from build123d import *

# Parameters (mm, degrees)
BOSS_EXTRUDE1_DEPTH = 4
SKETCH2_R           = 6.5
SKETCH2_R_2         = 2.25
SKETCH2_R_3         = 4
CUT_EXTRUDE1_DEPTH  = 4
BOSS_EXTRUDE2_START = 4
SKETCH3_R           = 22
SKETCH3_R_2         = 19
BOSS_EXTRUDE2_DEPTH = 15
SKETCH4_R           = 13.1
SKETCH4_R_2         = 11.1
BOSS_EXTRUDE3_DEPTH = 10
SKETCH5_R           = 1.5
CUT_EXTRUDE2_DEPTH  = 103.505675922
SKETCH6_W           = 10
SKETCH6_H           = 40
CUT_EXTRUDE3_DEPTH  = 103.505675922
FILLET1_R           = 2


with BuildPart() as part:
    # Sketch1 → Boss-Extrude1 (new body)
    with BuildSketch(Plane.XY):
        with BuildLine():
            Line((-14.334769336, 37.652327005), (51.395230664, 37.652327005))
            ThreePointArc((51.395230664, 37.652327005), (91.395230664, -2.347672995), (51.395230664, -42.347672995))
            Line((51.395230664, -42.347672995), (-14.334769336, -42.347672995))
            ThreePointArc((-14.334769336, -42.347672995), (-54.334769336, -2.347672995), (-14.334769336, 37.652327005))
        make_face()
    extrude(amount=BOSS_EXTRUDE1_DEPTH)

    # Sketch2 → Cut-Extrude1 (cut)
    with BuildSketch(Plane.XY):
        with Locations(Location((44.395230664, -2.347672995, 0), (0, 0, 180))):
            Circle(SKETCH2_R)
        with Locations(Location((51.395230664, 13.152327005, 0), (0, 0, 180))):
            Circle(SKETCH2_R_2)
        with Locations(Location((64.818624423, 5.402327005, 0), (0, 0, 180))):
            Circle(SKETCH2_R_2)
        with Locations(Location((64.818624423, -10.097672995, 0), (0, 0, 180))):
            Circle(SKETCH2_R_2)
        with Locations(Location((51.395230664, -17.847672995, 0), (0, 0, 180))):
            Circle(SKETCH2_R_2)
        with Locations(Location((37.971836906, -10.097672995, 0), (0, 0, 180))):
            Circle(SKETCH2_R_2)
        with Locations(Location((37.971836906, 5.402327005, 0), (0, 0, 180))):
            Circle(SKETCH2_R_2)
        with Locations(Location((-14.334769336, -2.347672995, 0), (0, 0, 180))):
            Circle(SKETCH2_R_3)
    extrude(amount=CUT_EXTRUDE1_DEPTH, mode=Mode.SUBTRACT)

    # Sketch3 → Boss-Extrude2 (add)
    with BuildSketch(Plane.XY.offset(BOSS_EXTRUDE2_START)):
        with Locations(Location((51.395230664, -2.347672995, 0), (0, 0, 180))):
            Circle(SKETCH3_R)
        with Locations(Location((51.395230664, -2.347672995, 0), (0, 0, 180))):
            Circle(SKETCH3_R_2, mode=Mode.SUBTRACT)
    extrude(amount=BOSS_EXTRUDE2_DEPTH)

    # Sketch4 → Boss-Extrude3 (add)
    with BuildSketch(Plane.XY):
        with Locations(Location((-14.334769336, -2.347672995, 0), (0, 0, 180))):
            Circle(SKETCH4_R)
        with Locations(Location((-14.334769336, -2.347672995, 0), (0, 0, 180))):
            Circle(SKETCH4_R_2, mode=Mode.SUBTRACT)
    extrude(amount=BOSS_EXTRUDE3_DEPTH)

    # Sketch5 → Cut-Extrude2 (cut, through all)
    with BuildSketch(Plane.XY):
        with Locations(Location((88.395230664, -2.347672995, 0), (0, 0, 180))):
            Circle(SKETCH5_R)
        with Locations(Location((-51.334769336, -2.347672995, 0), (0, 0, 180))):
            Circle(SKETCH5_R)
        with Locations(Location((51.395230664, 34.652327005, 0), (0, 0, 180))):
            Circle(SKETCH5_R)
        with Locations(Location((51.395230664, -39.347672995, 0), (0, 0, 180))):
            Circle(SKETCH5_R)
        with Locations(Location((-14.334769336, -39.347672995, 0), (0, 0, 180))):
            Circle(SKETCH5_R)
        with Locations(Location((-14.334769336, 34.652327005, 0), (0, 0, 180))):
            Circle(SKETCH5_R)
    extrude(amount=CUT_EXTRUDE2_DEPTH, mode=Mode.SUBTRACT)

    # Sketch6 → Cut-Extrude3 (cut, through all)
    with BuildSketch(Plane.XY):
        with Locations((18.530230664, 0)):
            Rectangle(SKETCH6_W, SKETCH6_H)
    extrude(amount=CUT_EXTRUDE3_DEPTH, mode=Mode.SUBTRACT)

    # Fillet1
    fillet1_edges = [part.edges().sort_by_distance(p)[0] for p in [
        (23.530230664, -20, 2),
        (23.530230664, 20, 2),
        (13.530230664, 20, 2),
        (13.530230664, -20, 2),
    ]]
    fillet(fillet1_edges, radius=FILLET1_R)


solid = part.part
The listing builds one solid part. Answer for the finished solid, in the listing's coordinates (mm). A direction names the side the tool comes from. Coordinates: 2 decimals unless noted, no trailing zeros. Loops run counter-clockwise (first coordinate to the right, second up) from the corner with the lowest first, then second, coordinate; pieces in that order, holes last. Notation, with made-up numbers: M 51,-10.5 L 81,-10.5 A21 cw 81,-5.5 Z; hole C 79,14.5 d11. An arc over 180 degrees is marked long. Answer in a Markdown table with one row per item.
1) Which of the six approach directions +Z, -Z, +X, -X, +Y, -Y give full straight-line access (tool end or side, diameter ignored) to faces 4 (the flat face through (-4.6, -8.2, 10)), 5 (the cylindrical face through (-3.939, 5.623, 6.958)), 6 (the flat face through (18, 20, 2)), 7 (the flat face through (3, -3, 0))?
Answers below:
| item | result |
|---|---|
| face 4 | +Z, -X, +Y, -Y |
| face 5 | +Z |
| face 6 | +Z, -Z |
| face 7 | -Z, +X, -X, +Y, -Y |
2) Determine the mould class of faces 1 (the cylindrical face through (62.74, -9.24, 1.97)), 2 (the cylindrical face through (-54.325, -3.227, 1.972)), 3 (the flat face through (3, -2, 4)) for opening direction Y: released by +Y, released by -Y, zero draft, split by the parting line, or undercut.
Answers below:
| item | result |
|---|---|
| face 1 | undercut |
| face 2 | split by the parting line |
| face 3 | zero draft |
3) Given pin 1 (6 mm diameter, centred on x = 9.5, z = 8, fed in from +Y); pin 2 (3.5 mm diameter, centred on x = 51.4, y = 34.65, fed in from +Z); pin 3 (8 mm diameter, centred on y = -13.5, z = 6.5, fed in from +X); pin 4 (21 mm diameter, centred on x = -14.5, y = 3.5, fed in from +Z), each flat-ended and moving along its own axis, determine where each tip first touches the part or whether it passes through.
Answers below:
| item | result |
|---|---|
| pin 1 | through |
| pin 2 | z = 4 |
| pin 3 | x = 90.58 |
| pin 4 | z = 10 |
4) Find section B-B (x = 61). Determine the outline of the cut face in (y, z), then the cut area to 3 significant figures.
Answers below:
| item | result |
|---|---|
| outline | M -41.18,0 L 36.48,0 L 36.48,4 L 17.44,4 L 17.44,19 L 14.05,19 L 14.05,4 L -18.74,4 L -18.74,19 L -22.14,19 L -22.14,4 L -41.18,4 Z |
| area | 413 mm^2 |
5) Find section C-C (z = 17.25). Determine the outline of the cut face in (x, y), then the cut area to 3 significant figures.
Answers below:
| item | result |
|---|---|
| outline | C 51.4,-2.35 d44; hole C 51.4,-2.35 d38 |
| area | 386 mm^2 |
6) Find the intervals of material crossed by probe 1 along X at (y, z) = (34.5, 3.5); probe 2 along Y at (x, z) = (51, 3.75); probe 3 along X at (y, z) = (3, 9.5), in increasing order.
Answers below:
| item | result |
|---|---|
| probe 1 | -29.9 to -15.83, -12.84 to 49.9, 52.89 to 66.96 |
| probe 2 | -42.35 to -40.79, -37.9 to -20.06, -15.63 to 10.94, 15.37 to 33.21, 36.1 to 37.65 |
| probe 3 | -26.29 to -24.06, -4.61 to -2.38, 30.06 to 33.16, 69.63 to 72.74 |
7) Find section D-D (y = -36). Determine the outline of the cut face in (x, z).
Answers below:
| item | result |
|---|---|
| outline | M -35.96,0 L 73.02,0 L 73.02,4 L -35.96,4 Z |
8) Find section A-A (z = 7.25). Determine the outline of the cut face in (x, y).
Answers below:
| item | result |
|---|---|
| outline | C -14.33,-2.35 d26.2; C 51.4,-2.35 d44; hole C -14.33,-2.35 d22.2; hole C 51.4,-2.35 d38 |
